Part model, mm, in its own coordinate system. A direction names the side the tool comes from. Coordinates: 2 decimals unless noted, no trailing zeros. Answer as a JSON object with one key per item and string values. Group by question number.
1. Drop flat-ended pins along their axis: pin 1 Ø1 at (x, z) = (159.5, -1.5) entering from -Y; pin 2 Ø2 at (x, z) = (168, -2) entering from +Y; pin 3 Ø6 at (x, y) = (301.5, -30) entering from +Z. Give the stop position or say it passes through.
2. Drill centre lines: L1, parallel to Y at x = 347, z = 2.25; L2, parallel to Y at x = 219, z = -0.75; L3, parallel to X at y = -34.5, z = -2.5. Where is each one in solid material? Low to high.
3. 3-axis set-ups, long thin cutter, end or side, ignore diameter. For faces 1 (the face through (467.753, -38.095, 0.044)), 2 (the face through (468.111, -49.878, 0.044)): which of +Z, -Z, +X, -X, +Y, -Y reach the whole face in a straight line?
from build123d import *

# Parameters (mm, degrees)
BOSS_EXTRUDE1_DEPTH = 3.175
CUT_EXTRUDE1_DEPTH  = 7.3500001
FILLET1_R           = 2.54
CUT_EXTRUDE2_DEPTH  = 7.62


with BuildPart() as part:
    # Sketch1 → Boss-Extrude1 (new body, symmetric)
    with BuildSketch(Plane.XY):
        with BuildLine():
            Line((499.61002795, -53.470702797), (1046.28548189, -53.470702797))
            add(Edge.make_bspline(
                [(2669.54, -9.569049356), (2615.393603553, -13.17073937), (2561.080658619, -16.536108081), (2506.205230446, -19.758621957), (2430.209106802, -23.505211705), (2354.212983157, -26.631486423), (2332.570330468, -27.480988169), (2156.268639429, -34.377768543), (1979.966947376, -41.628631248), (1824.114277635, -52.771265877), (1636.928606778, -53.579569849), (1449.742935921, -53.454024613), (1418.006730935, -53.470702797), (1324.899336146, -53.470702797), (1231.791940344, -53.470702797), (1170.441269319, -53.470702797), (1108.784075813, -53.470702797), (1047.126882346, -53.470702797), (1046.846414188, -53.470702797), (1046.565947184, -53.470702797), (1046.28548189, -53.470702797)],
                knots=[103.698913506, 103.698913506, 103.698913506, 103.698913506, 103.698913506, 103.698913506, 130.927896619, 130.927896619, 130.927896619, 141.337054719, 141.337054719, 141.337054719, 218.101815019, 218.101815019, 218.101815019, 233.772059419, 233.772059419, 233.772059419, 264.077723219, 264.077723219, 264.077723219, 264.2162088, 264.2162088, 264.2162088, 264.2162088, 264.2162088, 264.2162088], degree=5))
            Line((2669.54, -9.569049356), (2669.54, 9.5231025))
            add(Edge.make_bspline(
                [(2669.54, 9.5231025), (2667.126494524, 9.36235515), (2659.861586685, 8.880281494), (2635.666282302, 7.292469146), (2596.857665529, 4.826056853), (2545.729743039, 1.758344093), (2494.405305707, -1.098555235), (2451.533022267, -3.266573297), (2417.198316756, -4.86708361), (2391.457076919, -6.003589235), (2365.634736307, -7.086854581), (2339.546284672, -8.137729944), (2313.466132974, -9.165138371), (2287.612375486, -10.179478215), (2261.763347437, -11.201032297), (2227.285329715, -12.583842557), (2184.175569393, -14.36607236), (2132.429066114, -16.607427868), (2063.4255234, -19.708920485), (1977.174907635, -23.700543313), (1873.732451432, -28.149389221), (1770.37461881, -31.657468649), (1667.085687813, -33.793117556), (1581.011094491, -34.383188831), (1512.07397126, -34.4278026), (1443.061513477, -34.409510402), (1356.800927879, -34.424432812), (1218.794626954, -34.418464788), (1115.289022786, -34.420702797), (1046.28548189, -34.420702797)],
                knots=[103.571582669, 103.571582669, 103.571582669, 103.571582669, 104.300777207, 105.766098403, 110.877392287, 115.98868617, 121.099980054, 126.211273938, 128.76692088, 131.322567822, 133.878214764, 136.433861706, 138.989508647, 141.545155589, 144.100802531, 146.656449473, 151.767743357, 156.879037241, 161.990331124, 172.212918892, 182.43550666, 192.658094427, 202.880682195, 213.103269962, 218.214563846, 223.32585773, 233.548445497, 243.771033265, 264.2162088, 264.2162088, 264.2162088, 264.2162088], degree=3))
            Line((1046.28548189, -34.420702797), (499.61002795, -34.420702797))
            add(Edge.make_bspline(
                [(499.61002795, -34.420702797), (488.614737518, -34.420702797), (472.236395365, -34.420702798), (449.940231846, -34.420702794), (427.771305695, -34.42070281), (405.874681663, -34.420702712), (384.584909128, -34.420702942), (368.900229326, -34.420702244), (353.376568613, -34.420704862), (332.608466435, -34.420689186), (306.287754853, -34.420570006), (274.023487704, -34.420538256), (252.271015965, -34.420709741), (241.425150134, -34.420702761)],
                knots=[19.90682951, 19.90682951, 19.90682951, 19.90682951, 23.220120017, 24.876765271, 26.533410525, 29.846701033, 31.503346286, 33.15999154, 34.816636794, 36.473282048, 39.786572556, 43.099863063, 46.413153571, 46.413153571, 46.413153571, 46.413153571], degree=3))
            add(Edge.make_bspline(
                [(241.425150134, -34.420702761), (239.394928853, -34.420701455), (235.322322927, -34.420495867), (227.274423443, -34.398702533), (217.319360062, -34.297466855), (205.530690077, -33.976385563), (189.963341914, -33.212641271), (170.696984653, -31.543495194), (147.533261232, -28.314398128), (125.482753206, -24.202109872), (109.358914834, -20.622537553), (100.964116069, -18.612521054), (99.06, -18.149327722)],
                knots=[0, 0, 0, 0, 0.622088422, 1.244176844, 2.488353689, 3.732530533, 4.976707377, 7.465061066, 9.953414755, 12.441768444, 14.55823542, 15.180323842, 15.180323842, 15.180323842, 15.180323842], degree=3))
            Line((99.06, -18.149327722), (99.06, -37.741485304))
            add(Edge.make_bspline(
                [(241.425137875, -53.470702761), (224.286916993, -53.470691732), (207.149474967, -53.467315374), (190.203897513, -52.686577078), (161.734965878, -49.987457476), (133.266034188, -45.175583375), (121.749620566, -42.910592695), (110.349390726, -40.420274627), (99.06, -37.741485304)],
                knots=[0, 0, 0, 0, 0, 0, 8.71381608, 8.71381608, 8.71381608, 14.701907176, 14.701907176, 14.701907176, 14.701907176, 14.701907176, 14.701907176], degree=5))
            add(Edge.make_bspline(
                [(499.61002795, -53.470702797), (492.136820835, -53.470702797), (484.754348064, -53.470702797), (477.443025859, -53.470702797), (448.516583145, -53.470702797), (419.590140517, -53.470702797), (398.368118521, -53.470702797), (355.647540186, -53.470702797), (312.926961851, -53.470702797), (289.235090436, -53.470293029), (265.364963651, -53.470705034), (241.4948369, -53.470702789), (241.471603891, -53.470702785), (241.448370882, -53.470702776), (241.425137875, -53.470702761)],
                knots=[19.90682951, 19.90682951, 19.90682951, 19.90682951, 19.90682951, 19.90682951, 23.637897311, 23.637897311, 23.637897311, 34.276545571, 34.276545571, 34.276545571, 46.401340901, 46.401340901, 46.401340901, 46.413153571, 46.413153571, 46.413153571, 46.413153571, 46.413153571, 46.413153571], degree=5))
        make_face()
    extrude(amount=BOSS_EXTRUDE1_DEPTH, both=True)

    # Sketch2 → Cut-Extrude1 (cut, through all)
    with BuildSketch(Plane.XY.offset(3.175)):
        with BuildLine():
            add(Edge.make_bspline(
                [(2312.9875, -9.183260037), (2304.505441691, -9.516700376), (2287.441020622, -10.186250162), (2261.763347437, -11.201032297), (2228.230552004, -12.545932515), (2203.310445107, -13.575047161), (2187.00995947, -14.263260037)],
                knots=[139.04033329, 139.04033329, 139.04033329, 139.04033329, 141.545155589, 144.100802531, 146.656449473, 151.487488909, 151.487488909, 151.487488909, 151.487488909], degree=3))
            Line((2187.00995947, -14.263260037), (2312.9875, -14.263260037))
            Line((2312.9875, -14.263260037), (2312.9875, -9.183260037))
        make_face()
    extrude(amount=-CUT_EXTRUDE1_DEPTH, mode=Mode.SUBTRACT)

    # Fillet1
    fillet1_edges = [part.edges().sort_by_distance(p)[0] for p in [
        (2669.54, -9.569049356, -1.5875),
        (2669.54, 9.5231025, -1.5875),
        (99.06, -37.741485304, -1.5875),
        (99.06, -18.149327722, -1.5875),
        (2312.9875, -9.183260037, 1.5875),
        (2312.9875, -14.263260037, 0),
    ]]
    fillet(fillet1_edges, radius=FILLET1_R)

    # Sketch3 → Cut-Extrude2 (cut)
    with BuildSketch(Plane.XY.offset(3.175)):
        Polygon((463.358597157, -34.420702797), (472.271656585, -41.874419167), (463.358597157, -46.384200616), (472.997412797, -53.470702797), (510.09583662, -269.844988776), (2795.524214409, -269.844988776), (2811.168313051, 250.910269335), (463.358597157, 321.441226467), align=None)
    extrude(amount=-CUT_EXTRUDE2_DEPTH, mode=Mode.SUBTRACT)


solid = part.part
Outcome:
{
 "1": {"pin 1": "stops at y = -49.22", "pin 2": "stops at y = -30.91", "pin 3": "passes through"},
 "2": {"L1": "y = -53.47 to -34.42", "L2": "y = -53.35 to -34.29", "L3": "x = 99.06 to 463.45"},
 "3": {"face 1": "+Z, -Z, +X, +Y", "face 2": "+Z, -Z, +X"}
}
